Part print with two shaded views. Sizes in mm from the minimum x, y, z corner. A direction names the side the tool comes from. Coordinates: 2 decimals unless noted, no trailing zeros. Order: outer loops, then holes, each group sorted by start corner. A loop starts at its lowest first (then second) coordinate and runs counter-clockwise, first axis right, second up. Notation, with made-up numbers: (-25.75, -36) - (20.25, -36) arc R25 ccw to (20.25, -1) - close; hole circle Ø1 at (-13.75, 43.5). An arc over 180 degrees is marked (long way). Write each question's results on one line, items separated by ' | '. Start each with the question number.
Q1. Band-saw the part on A-A, the plane x = 5.75. Write the cut outline in (y, z) (1 decimal).
Q2. Pin check, flat tips, straight feed: P1, Ø1.2, axis at x = 7, y = 7.5, coming from the -Z side; P2, Ø3, axis at y = 2.5, z = 14, coming from the -X side (1 decimal); P3, Ø5, axis at x = 5.5, z = 15, coming from the -Y side (1 decimal); P4, Ø6, axis at x = 10.5, y = 7, coming from the -Z side. Stop position of each tip, or through.
Q3. Band-saw the part on C-C, the plane y = 8.75. Write the cut outline in (x, z).
Q4. Band-saw the part on D-D, the plane x = 10.25. Write the cut outline in (y, z).
Q5. Which spindle directions (+Z, -Z, +X, -X, +Y, -Y) get a long thin tool onto all of the face, cutting with end or side? Do the marked faces 1, 2 and 3. Say none if no direction does.
Q6. Wall check: probe 1 along Z at (x, y) = (8.5, 7.75); probe 2 along X at (y, z) = (4.5, 13.25); probe 3 along Z at (x, y) = (7.5, 0.5). Give the ranges that are in metal, low to high.
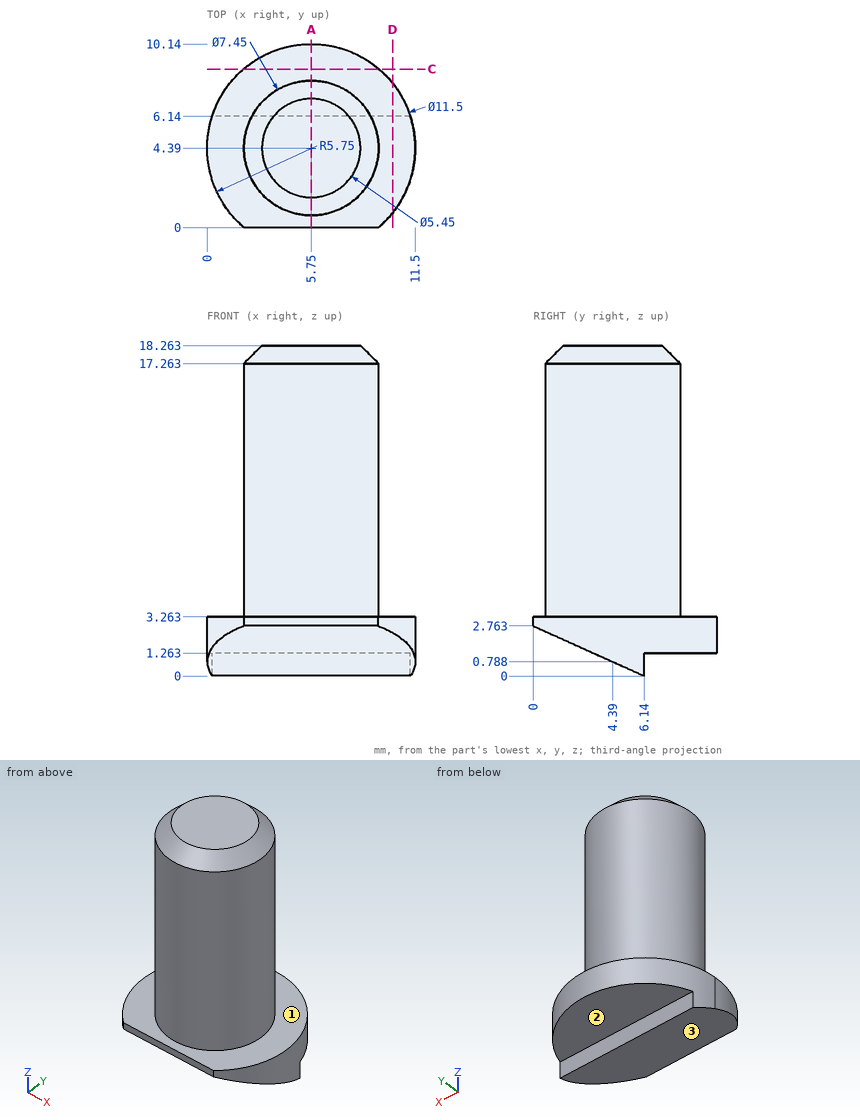
Results below:
1) outline: (0, 2.8) - (6.1, 0) - (6.1, 1.3) - (10.1, 1.3) - (10.1, 3.3) - (8.1, 3.3) - (8.1, 17.3) - (7.1, 18.3) - (1.7, 18.3) - (0.7, 17.3) - (0.7, 3.3) - (0, 3.3) - close
2) P1: stops at z = 1.26 | P2: stops at x = 2 | P3: stops at y = 0.7 | P4: stops at z = 0
3) outline: (2, 1.26) - (9.5, 1.26) - (9.5, 3.26) - (2, 3.26) - close
4) outline: (0.81, 2.4) - (6.14, 0) - (6.14, 1.26) - (7.97, 1.26) - (7.97, 3.26) - (0.81, 3.26) - close
5) face 1: +Z | face 2: -Z, +X, -X, +Y | face 3: -Z, +X, -X, -Y
6) probe 1: z = 1.26 to 3.26 | probe 2: x = 2.03 to 9.47 | probe 3: z = 2.54 to 3.26
